For this review, take the finished solid that the model builds, in its own axes (mm). A direction names the side the tool comes from. Give positions to 0.01 mm unless a question says otherwise; leave off trailing zeros. Order: outer loops, then holes, each group sorted by start corner. A loop starts at its lowest first (then second) coordinate and runs counter-clockwise, first axis right, second up.
Item 1: For probe 1 along X at (y, z) = (3.75, 0.45); probe 2 along Y at (x, z) = (90.9, 1.5); probe 3 along Y at (x, z) = (85, 1.95), list the stretches that pass through material, from the lowest coordinate up.
Item 2: For P1, Ø3.5, axis at x = 5.1, y = 3.75, coming from the +Z side, flat-tipped, find the tip position at first contact; note if it passes through.
Item 3: Consider section C-C (y = 8). Give the boundary of the cut face in (x, z).
Item 4: Consider section D-D (x = 36). Give the boundary of the cut face in (y, z), plus the area to 3 significant figures.
Item 5: Consider section A-A (x = 5.1). Give the boundary of the cut face in (y, z).
Item 6: Machinability: for faces 1 (the flat face through (72.4, 32, 1)), 2 (the flat face through (47, 0, 1)), which of the approach directions +Z, -Z, +X, -X, +Y, -Y give a long, thin tool a straight path to every point of the face, cutting with its end or side? Answer none if there is none.
Item 7: The part is to be moulded in two halves that separate along X. For faces 3 (the flat face through (81, 19.25, 1)), 4 (the flat face through (80, 40.75, 1)), 5 (the flat face through (49, 46, 1)), 6 (the flat face through (96, 23, 1)), say which applies: released by +X, released by -X, zero draft, split by the parting line, or undercut.
Item 8: Consider section B-B (z = 1.65). Give the boundary of the cut face in (x, y), plus the area to 3 significant figures.
Autodesk Fusion 360 part; units mm, degrees
sketch "Sketch1" plane through (0, 0, 0) normal (0, 0, 1) x (1, 0, 0)
  line L0 (0, 0) -> (96, 0)
  line L1 (96, 0) -> (96, 46)
  line L2 (96, 46) -> (0, 46)
  line L3 (0, 46) -> (0, 0)
  dimension "d1" = 96
  dimension "d2" = 46
extrude "Extrude1" add sketch "Sketch1" along normal blind 2
fillet "Fillet1" radius 1 4 edges at (96, 0, 1) (96, 46, 1) (0, 46, 1) (0, 0, 1)
sketch "Sketch2" plane through (0, 0, 2) normal (0, 0, 1) x (-1, 0, 0)
  arc A0 (0, -1) -> (-1, 0) centre (-1, -1) ccw
  line L0 (-1, 0) -> (-95, 0)
  arc A1 (-95, 0) -> (-96, -1) centre (-95, -1) ccw
  line L1 (-96, -1) -> (-96, -45)
  arc A2 (-96, -45) -> (-95, -46) centre (-95, -45) ccw
  line L2 (-95, -46) -> (-1, -46)
  arc A3 (-1, -46) -> (0, -45) centre (-1, -45) ccw
  line L3 (0, -45) -> (0, -1)
  circle A4 centre (-5.1, -42.25) radius 1.6
  circle A5 centre (-90.9, -42.25) radius 1.6
  circle A6 centre (-90.9, -3.75) radius 1.6
  circle A7 centre (-5.1, -3.75) radius 1.6
  dimension "d7" = 3.2
  dimension "d8" = 3.75
  dimension "d9" = 5.1
  dimension "d10" = 3.2
  dimension "d11" = 3.2
  dimension "d12" = 3.2
  dimension "d13" = 3.75
  dimension "d14" = 5.1
  dimension "d15" = 3.75
  dimension "d16" = 5.1
  dimension "d17" = 5.1
  dimension "d18" = 3.75
extrude "Extrude2" cut sketch "Sketch2" against normal blind 2 contours A4 | A5 | A6 | A7
sketch "Sketch3" plane through (0, 0, 2) normal (0, 0, 1) x (-1, 0, 0)
  circle A0 centre (-90.9, -3.75) radius 1.6
  circle A1 centre (-5.1, -3.75) radius 1.6
  circle A2 centre (-90.9, -42.25) radius 1.6
  circle A3 centre (-5.1, -42.25) radius 1.6
  arc A4 (0, -1) -> (-1, 0) centre (-1, -1) ccw
  line L0 (-1, 0) -> (-95, 0)
  arc A5 (-95, 0) -> (-96, -1) centre (-95, -1) ccw
  line L1 (-96, -1) -> (-96, -45)
  arc A6 (-96, -45) -> (-95, -46) centre (-95, -45) ccw
  line L2 (-95, -46) -> (-1, -46)
  arc A7 (-1, -46) -> (0, -45) centre (-1, -45) ccw
  line L3 (0, -45) -> (0, -1)
  line L4 (-2.5, -46) -> (-2.5, 0) construction
  line L5 (-7.3, -46) -> (-7.3, 0)
  line L6 (-93.5, -46) -> (-93.5, 0)
  line L7 (-88.5, -46) -> (-88.5, 0)
  line L8 (-7.3, -44.75) -> (-67.5, -44.75)
  line L9 (-67.5, -44.75) -> (-67.5, -0.75)
  line L10 (-67.5, -0.75) -> (-7.3, -0.75)
  line L11 (-7.3, -0.75) -> (-7.3, -44.75)
  line L12 (0, -23) -> (-96, -23) construction
  dimension "d21" = 2.6
  dimension "d22" = 4.8
  dimension "d23" = 2.6
  dimension "d24" = 5
  dimension "d26" = 44
  dimension "d27" = 44
  dimension "d29" = 21.75
  dimension "d30" = 22
  dimension "d31" = 4.8
  dimension "d32" = 21
  dimension "d34" = 60.2
extrude "Extrude3" cut sketch "Sketch3" against normal blind 2 contours L5 L8 L9 L10 L11
sketch "Sketch4" plane through (0, 0, 2) normal (0, 0, 1) x (-1, 0, 0)
  line L0 (-67.5, -44.75) -> (-67.5, -0.75)
  line L1 (-67.5, -0.75) -> (-7.3, -0.75)
  line L2 (-7.3, -0.75) -> (-7.3, -44.75)
  line L3 (-7.3, -44.75) -> (-67.5, -44.75)
  circle A0 centre (-90.9, -3.75) radius 1.6
  circle A1 centre (-5.1, -3.75) radius 1.6
  circle A2 centre (-90.9, -42.25) radius 1.6
  circle A3 centre (-5.1, -42.25) radius 1.6
  arc A4 (0, -1) -> (-1, 0) centre (-1, -1) ccw
  line L4 (-1, 0) -> (-95, 0)
  arc A5 (-95, 0) -> (-96, -1) centre (-95, -1) ccw
  line L5 (-96, -1) -> (-96, -45)
  arc A6 (-96, -45) -> (-95, -46) centre (-95, -45) ccw
  line L6 (-95, -46) -> (-1, -46)
  arc A7 (-1, -46) -> (0, -45) centre (-1, -45) ccw
  line L7 (0, -45) -> (0, -1)
  line L8 (-93.5, -46) -> (-93.5, 0)
  line L9 (-88.5, -46) -> (-88.5, 0)
  line L10 (-73.4, -39.75) -> (-87.8, -39.75)
  line L11 (-87.8, -39.75) -> (-87.8, -25.35)
  line L12 (-87.8, -25.35) -> (-73.4, -25.35)
  line L13 (-73.4, -25.35) -> (-73.4, -39.75)
  line L14 (-74.6, -18.25) -> (-86.6, -18.25)
  line L15 (-86.6, -18.25) -> (-86.6, -6.25)
  line L16 (-86.6, -6.25) -> (-74.6, -6.25)
  line L17 (-74.6, -6.25) -> (-74.6, -18.25)
  line L18 (-72.4, -40.75) -> (-88.8, -40.75)
  line L19 (-88.8, -40.75) -> (-88.8, -24.35)
  line L20 (-88.8, -24.35) -> (-72.4, -24.35)
  line L21 (-72.4, -24.35) -> (-72.4, -40.75)
  line L22 (-73.6, -5.25) -> (-73.6, -19.25)
  line L23 (-73.6, -19.25) -> (-87.6, -19.25)
  line L24 (-87.6, -19.25) -> (-87.6, -5.25)
  line L25 (-87.6, -5.25) -> (-73.6, -5.25)
  dimension "d38" = 2.6
  dimension "d39" = 5
  dimension "d40" = 14.4
  dimension "d41" = 14.4
  dimension "d42" = 5.7
  dimension "d44" = 12
  dimension "d45" = 12
  dimension "d46" = 6.9
  dimension "d47" = 7.1
  dimension "d48" = -1
  dimension "d49" = -1
  dimension "d50" = 5
extrude "Extrude4" cut sketch "Sketch4" against normal blind 2 contours L9 L18 L20 L21 | L10 L11 L12 L13 | L14 L15 L16 L17 | L22 L23 L24 L25
sketch "Sketch5" plane through (0, 0, 2) normal (0, 0, 1) x (-1, 0, 0)
  line L0 (-88.5, -40.75) -> (-88.5, -24.35)
  line L1 (-88.5, -24.35) -> (-72.4, -24.35)
  line L2 (-72.4, -24.35) -> (-72.4, -40.75)
  line L3 (-72.4, -40.75) -> (-88.5, -40.75)
  line L4 (-73.6, -19.25) -> (-87.6, -19.25)
  line L5 (-87.6, -19.25) -> (-87.6, -5.25)
  line L6 (-87.6, -5.25) -> (-73.6, -5.25)
  line L7 (-73.6, -5.25) -> (-73.6, -19.25)
  line L8 (-67.5, -44.75) -> (-67.5, -0.75)
  line L9 (-67.5, -0.75) -> (-7.3, -0.75)
  line L10 (-7.3, -0.75) -> (-7.3, -44.75)
  line L11 (-7.3, -44.75) -> (-67.5, -44.75)
  circle A0 centre (-90.9, -3.75) radius 1.6
  circle A1 centre (-5.1, -3.75) radius 1.6
  circle A2 centre (-90.9, -42.25) radius 1.6
  circle A3 centre (-5.1, -42.25) radius 1.6
  arc A4 (0, -1) -> (-1, 0) centre (-1, -1) ccw
  line L12 (-1, 0) -> (-95, 0)
  arc A5 (-95, 0) -> (-96, -1) centre (-95, -1) ccw
  line L13 (-96, -1) -> (-96, -45)
  arc A6 (-96, -45) -> (-95, -46) centre (-95, -45) ccw
  line L14 (-95, -46) -> (-1, -46)
  arc A7 (-1, -46) -> (0, -45) centre (-1, -45) ccw
  line L15 (0, -45) -> (0, -1)
  dimension "d53" = 3.75
  dimension "d54" = 3.75
  dimension "d55" = 3.75
equation "d21 = 1 mm + ( ( 3.2 / 2 ) * 1 mm )"
equation "d29 = ( 43.5 / 2 ) * 1 mm"
equation "d38 = ( 3.2 / 2 ) * 1 mm + 1 mm"
Resolved:
1. probe 1: x = 0 to 3.5, 6.7 to 7.3, 67.5 to 89.3, 92.5 to 96
1. probe 2: y = 0 to 2.15, 5.35 to 40.65, 43.85 to 46
1. probe 3: y = 0 to 5.25, 19.25 to 24.35, 40.75 to 46
2. P1: stops at z = 2
3. outline: (0, 0) - (7.3, 0) - (7.3, 2) - (0, 2) - close; (67.5, 0) - (73.6, 0) - (73.6, 2) - (67.5, 2) - close; (87.6, 0) - (96, 0) - (96, 2) - (87.6, 2) - close
4. outline: (0, 0) - (0.75, 0) - (0.75, 2) - (0, 2) - close; (44.75, 0) - (46, 0) - (46, 2) - (44.75, 2) - close
4. area: 4.00 mm2
5. outline: (0, 0) - (2.15, 0) - (2.15, 2) - (0, 2) - close; (5.35, 0) - (40.65, 0) - (40.65, 2) - (5.35, 2) - close; (43.85, 0) - (46, 0) - (46, 2) - (43.85, 2) - close
6. face 1: +Z, -Z
6. face 2: +Z, -Z, +X, -X, -Y
7. face 3: undercut
7. face 4: undercut
7. face 5: zero draft
7. face 6: released by +X
8. outline: (0, 1) arc R1 ccw to (1, 0) - (95, 0) arc R1 ccw to (96, 1) - (96, 45) arc R1 ccw to (95, 46) - (1, 46) arc R1 ccw to (0, 45) - close; hole circle Ø3.2 at (5.1, 3.75); hole circle Ø3.2 at (5.1, 42.25); hole (7.3, 0.75) - (67.5, 0.75) - (67.5, 44.75) - (7.3, 44.75) - close; hole (72.4, 24.35) - (88.5, 24.35) - (88.5, 40.75) - (72.4, 40.75) - close; hole (73.6, 5.25) - (87.6, 5.25) - (87.6, 19.25) - (73.6, 19.25) - close; hole circle Ø3.2 at (90.9, 3.75); hole circle Ø3.2 at (90.9, 42.25)
8. area: 1,270 mm2
